from build123d import *

# Parameters (mm, degrees)
EXTRUDE1_DEPTH     = 40
CUT_EXTRUDE1_DEPTH = 126.980762114
EXTRUDE2_DEPTH     = 70
EXTRUDE3_DEPTH     = 70


with BuildPart() as part:
    # Sketch1 → Extrude1 (new body)
    with BuildSketch(Plane(origin=(0, 0, 0), x_dir=(1, 0, 0), z_dir=(0, 1, 0))):
        Polygon((0, 0), (50, 86.602540378), (-1.961524227, 116.602540378), (-51.961524227, 30), align=None)
    extrude(amount=EXTRUDE1_DEPTH)

    # Sketch2 → Cut-Extrude1 (cut, through all)
    with BuildSketch(Plane(origin=(0, 0, 0), x_dir=(0.866025404, 0, 0.5), z_dir=(-0.5, 0, 0.866025404))):
        Polygon((0, 20), (-60, 40), (0, 40), align=None)
    extrude(amount=-CUT_EXTRUDE1_DEPTH, mode=Mode.SUBTRACT)

    # Sketch3 → Extrude2 (add)
    with BuildSketch(Plane(origin=(0, 0, 0), x_dir=(1, 0, 0), z_dir=(0, 1, 0))):
        Polygon((-65.442286341, 66.650635095), (-40.442286341, 109.951905284), (20.179491924, 74.951905284), (-4.820508076, 31.650635095), align=None)
    extrude(amount=EXTRUDE2_DEPTH)

    # Sketch4 → Extrude3 (add)
    with BuildSketch(Plane(origin=(-17.320508076, 0, -10), x_dir=(0.5, 0, -0.866025404), z_dir=(0.866025404, 0, 0.5))):
        Polygon((25, 70), (75, 70), (50, 95), align=None)
    extrude(amount=-EXTRUDE3_DEPTH)


solid = part.part
The model under review builds one solid part; all positions refer to its coordinate system, in mm. A direction names the side the tool comes from. Round coordinates to 2 decimals unless told otherwise and drop trailing zeros. Write each loop counter-clockwise with the first axis right and the second up, starting at its lowest first coordinate (ties: lowest second). Pieces come first, ordered by that corner, then holes. Notation, with made-up numbers: (4.25, 89) - (46.25, 89) arc R25 ccw to (46.25, 103) - close; hole circle Ø4 at (78, 46). An arc over 180 degrees is marked (long way). One line per item, written item: value. Start each with the question number.
1. Consider section D-D on x = -8.5. Write out the cut boundary in (y, z) (1 decimal), and give its area (3 significant figures).
2. Consider section B-B on x = -42. Write out the cut boundary in (y, z), and give its area (3 significant figures).
3. To check wall thickness, follow L1, parallel to Z at x = -41, y = 35; L2, parallel to Z at x = -51.5, y = 21.5; L3, parallel to X at y = 19, z = -93. State the ranges of each line that lie inside material, in increasing order. Write a range as from..to.
4. Machinability: for faces 1 (the face through (-45.62, 19.72, -40.98)), 2 (the face through (24.65, 9.86, -42.695)), which of the approach directions +Z, -Z, +X, -X, +Y, -Y give a long, thin tool a straight path to every point of the face, cutting with its end or side? Answer none if there is none.
5. Clearance check with flat-ended pins moving along their axes: P1, Ø2, axis at x = -23, y = 78, coming from the +Z side; P2, Ø2, axis at y = 70, z = -62, coming from the +X side; P3, Ø2, axis at x = -28.5, z = -66, coming from the +Y side. State where each tip first meets the part, or that it passes through.
6. The part is to be moulded in two halves that separate along X. For faces 3 (the face through (-17.292, 42.288, -96.586)), 4 (the face through (-7, 0, -59)), 5 (the face through (-15.87, 82.325, -81.533)), 6 (the face through (-8.124, 19.72, -105.929)), say which applies: released by +X, released by -X, zero draft, split by the parting line, or undercut.
7. Consider section A-A on y = 8. Write out the cut boundary in (x, z), and give its area (3 significant figures).
8. Consider section C-C on z = -105. Write out the cut boundary in (x, y).
Checks:
1. outline: (0, -105.3) - (40, -105.3) - (37.7, -91.5) - (70, -91.5) - (95, -62.6) - (70, -33.8) - (28.1, -33.8) - (23.3, -4.9) - (0, -4.9) - close
1. area: 6,040 mm^2
2. outline: (0, -107.25) - (73.12, -107.25) - (95, -81.98) - (70, -53.12) - (0, -53.12) - close; (0, -47.25) - (40, -47.25) - (36.17, -24.25) - (0, -24.25) - close
2. area: 5,380 mm^2
3. L1: z = -108.99..-52.54, -48.99..-23.67
3. L2: z = -90.8..-58.6, -30.8..-29.73
3. L3: x = -50.23..38.92
4. face 1: -X, +Y, -Y
4. face 2: +Z, +X, +Y, -Y
5. P1: stops at z = -50.09
5. P2: stops at x = 13.28
5. P3: stops at y = 88.91
6. face 3: undercut
6. face 4: zero draft
6. face 5: released by +X
6. face 6: undercut
7. outline: (-65.44, -66.65) - (-40.44, -109.95) - (-14.46, -94.95) - (-1.96, -116.6) - (50, -86.6) - (0, 0) - (-51.96, -30) - (-39.46, -51.65) - close
7. area: 7,500 mm^2
8. outline: (-43.3, 0) - (-31.87, 0) - (-31.87, 70) - (-43.3, 75.72) - close; (-8.66, 0) - (18.13, 0) - (18.13, 32.26) - (-8.66, 40) - close
